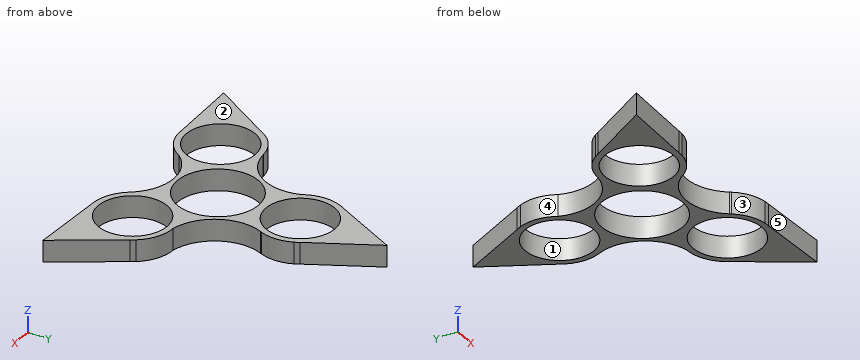
```python
from build123d import *

# Parameters (mm, degrees)
F0_R     = 11.2
F0_R_2   = 13.2
F1_DEPTH = 7


with BuildPart() as f1:
    # F0 (on Top) → F1 (new body)
    with BuildSketch(Plane.XY):
        with BuildLine():
            ThreePointArc((12.100793, 21.66292), (11.990187, 21.427431), (11.883555, 21.190116))
            ThreePointArc((11.883555, 21.190116), (11.994504, 21.425448), (12.100793, 21.66292))
        make_face()
        with BuildLine():
            ThreePointArc((23.327707, -0.268258), (12.397461, 7.683314), (11.883555, 21.190116))
            ThreePointArc((11.883555, 21.190116), (11.990187, 21.427431), (12.100793, 21.66292))
            ThreePointArc((12.100793, 21.66292), (13.199904, 26.986831), (12.060238, 32.302209))
            Line((12.060238, 32.302209), (11.254453, 33.834145))
            ThreePointArc((11.254453, 33.834145), (0, 40.136516), (-11.254453, 33.834145))
            Line((-11.254453, 33.834145), (-12.060238, 32.302209))
            ThreePointArc((-12.060238, 32.302209), (-13.181817, 26.243916), (-11.431535, 20.336516))
            ThreePointArc((-11.431535, 20.336516), (-12.852676, 6.894859), (-24.292957, -0.303597))
            ThreePointArc((-24.292957, -0.303597), (-24.551793, -0.329909), (-24.811035, -0.351866))
            ThreePointArc((-24.811035, -0.351866), (-29.971233, -2.061963), (-34.004652, -5.706632))
            Line((-34.004652, -5.706632), (-34.928456, -7.17043))
            ThreePointArc((-34.928456, -7.17043), (-34.759243, -20.068258), (-23.674002, -26.663715))
            Line((-23.674002, -26.663715), (-21.944414, -26.595577))
            ThreePointArc((-21.944414, -26.595577), (-16.136989, -24.537746), (-11.896172, -20.068258))
            ThreePointArc((-11.896172, -20.068258), (0.455215, -14.578173), (12.409401, -20.886519))
            ThreePointArc((12.409401, -20.886519), (12.561606, -21.097522), (12.710243, -21.311054))
            ThreePointArc((12.710243, -21.311054), (16.771329, -24.924868), (21.944414, -26.595577))
            Line((21.944414, -26.595577), (23.674002, -26.663715))
            ThreePointArc((23.674002, -26.663715), (34.759243, -20.068258), (34.928456, -7.17043))
            Line((34.928456, -7.17043), (34.004652, -5.706632))
            ThreePointArc((34.004652, -5.706632), (29.318806, -1.706169), (23.327707, -0.268258))
        make_face()
        with Locations((-23.327707, -13.468258)):
            Circle(F0_R, mode=Mode.SUBTRACT)
        with Locations((23.327707, -13.468258)):
            Circle(F0_R, mode=Mode.SUBTRACT)
        Circle(F0_R_2, mode=Mode.SUBTRACT)
        with Locations((0, 26.936516)):
            Circle(F0_R, mode=Mode.SUBTRACT)
        with BuildLine():
            Line((11.254453, 33.834145), (12.060238, 32.302209))
            ThreePointArc((12.060238, 32.302209), (11.682483, 33.081399), (11.254453, 33.834145))
        make_face()
        with BuildLine():
            ThreePointArc((34.928456, -7.17043), (34.490574, -6.423372), (34.004652, -5.706632))
            Line((34.004652, -5.706632), (34.928456, -7.17043))
        make_face()
        with BuildLine():
            ThreePointArc((-11.254453, 33.834145), (0, 40.136516), (11.254453, 33.834145))
            Line((11.254453, 33.834145), (0, 55.230804))
            Line((0, 55.230804), (-11.254453, 33.834145))
        make_face()
        with BuildLine():
            Line((47.831279, -27.615402), (34.928456, -7.17043))
            ThreePointArc((34.928456, -7.17043), (34.759243, -20.068258), (23.674002, -26.663715))
            Line((23.674002, -26.663715), (47.831279, -27.615402))
        make_face()
        with BuildLine():
            Line((-12.060238, 32.302209), (-11.254453, 33.834145))
            ThreePointArc((-11.254453, 33.834145), (-11.682483, 33.081399), (-12.060238, 32.302209))
        make_face()
        with BuildLine():
            ThreePointArc((21.944414, -26.595577), (22.80809, -26.658027), (23.674002, -26.663715))
            Line((23.674002, -26.663715), (21.944414, -26.595577))
        make_face()
        with BuildLine():
            ThreePointArc((12.409401, -20.886519), (12.55773, -21.100269), (12.710243, -21.311054))
            ThreePointArc((12.710243, -21.311054), (12.561606, -21.097522), (12.409401, -20.886519))
        make_face()
        with BuildLine():
            ThreePointArc((-24.811035, -0.351866), (-24.551793, -0.329909), (-24.292957, -0.303597))
            ThreePointArc((-24.292957, -0.303597), (-24.552234, -0.325179), (-24.811035, -0.351866))
        make_face()
        with BuildLine():
            Line((-34.928456, -7.17043), (-34.004652, -5.706632))
            ThreePointArc((-34.004652, -5.706632), (-34.490574, -6.423372), (-34.928456, -7.17043))
        make_face()
        with BuildLine():
            ThreePointArc((-23.674002, -26.663715), (-22.80809, -26.658027), (-21.944414, -26.595577))
            Line((-21.944414, -26.595577), (-23.674002, -26.663715))
        make_face()
        with BuildLine():
            ThreePointArc((-23.674002, -26.663715), (-34.759243, -20.068258), (-34.928456, -7.17043))
            Line((-34.928456, -7.17043), (-47.831279, -27.615402))
            Line((-47.831279, -27.615402), (-23.674002, -26.663715))
        make_face()
    extrude(amount=F1_DEPTH)


solid = f1.part
```
Could you check a few things on this model? Use its own coordinates, in mm. Face numbers are marked on the shaded views. A direction names the side the tool comes from. Coordinates: 2 decimals unless noted, no trailing zeros. Write each loop counter-clockwise with the first axis right and the second up, starting at its lowest first coordinate (ties: lowest second). Pieces come first, ordered by that corner, then holes. Notation, with made-up numbers: (22.5, 49.25) -> (44.5, 49.25) arc R13 ccw to (44.5, 58.25) -> close; hole circle Ø1 at (7.25, 79). An arc over 180 degrees is marked (long way). Write item = value, one per line. Start each with the question number.
(1) I want a section at A-A (x = -16.5). Please give me the cut outline in (y, z).
(2) I want a section at C-C (z = 4). Please give me the cut outline in (x, y).
(3) I need wall thicknesses on line 1 (X direction, y = -23.5, z = 5.5); line 2 (X direction, y = 20, z = 6.75); line 3 (X direction, y = 33, z = 4). Which ranges of each line are inside material? Lowest first, please. Write a range as [from, to].
(4) I want a section at B-B (y = 9). Please give me the cut outline in (x, z), plus the area to 3 significant figures.
(5) Which directions (+Z, -Z, +X, -X, +Y, -Y) give clear straight access to the entire face, cutting with the end or side of a thin tool? Please do the marked faces 4 and 5.
(6) We'd pull the mould along Y, two halves only. Please class the marked faces 1, 2 and 3: released by +Y, released by -Y, zero draft, split by the parting line, or undercut.
(7) Will these pins go through, and if not, where does the flat tip stop? pin 1 (1.5 mm diameter, centred on x = 35, z = 3.5, fed in from -Y); pin 2 (3 mm diameter, centred on x = 23.5, z = 3, fed in from +Y); pin 3 (2 mm diameter, centred on y = -1, z = 3, fed in from -X); pin 4 (13.5 mm diameter, centred on x = -23.33, y = -13.47, fed in from +Z).
(8) I want a section at D-D (x = -1.5). Please give me the cut outline in (y, z).
Result set:
q1.outline = (-24.77, 0) -> (-22.35, 0) -> (-22.35, 7) -> (-24.77, 7) -> close; (-4.59, 0) -> (2.85, 0) -> (2.85, 7) -> (-4.59, 7) -> close
q2.outline = (-47.83, -27.62) -> (-23.67, -26.66) arc R13.2 ccw to (-21.94, -26.6) arc R13.2 ccw to (-11.9, -20.07) arc R15.48 cw to (12.41, -20.89) arc R13.2 ccw to (12.71, -21.31) arc R13.2 ccw to (21.94, -26.6) arc R13.2 ccw to (23.67, -26.66) -> (47.83, -27.62) -> (34.93, -7.17) arc R13.2 ccw to (34, -5.71) arc R13.2 ccw to (23.33, -0.27) arc R15.48 cw to (11.88, 21.19) arc R13.2 ccw to (12.1, 21.66) arc R13.2 ccw to (12.06, 32.3) arc R13.2 ccw to (11.25, 33.83) -> (0, 55.23) -> (-11.25, 33.83) arc R13.2 ccw to (-12.06, 32.3) arc R13.2 ccw to (-11.43, 20.34) arc R15.48 cw to (-24.29, -0.3) arc R13.2 ccw to (-24.81, -0.35) arc R13.2 ccw to (-34, -5.71) arc R13.2 ccw to (-34.93, -7.17) -> close; hole circle Ø22.4 at (-23.33, -13.47); hole circle Ø26.4 at (0, 0); hole circle Ø22.4 at (0, 26.94); hole circle Ø22.4 at (23.33, -13.47)
q3.line_1 = [-45.23, -28.31], [-18.35, -14.75], [14.75, 18.35], [28.31, 45.23]
q3.line_2 = [-11.31, -8.79], [8.79, 11.42]
q3.line_3 = [-11.72, -9.42], [9.42, 11.72]
q4.outline = (-11.76, 0) -> (-9.66, 0) -> (-9.66, 7) -> (-11.76, 7) -> close; (9.66, 0) -> (11.77, 0) -> (11.77, 7) -> (9.66, 7) -> close
q4.area = 29.5 mm2
q5.face_4 = +Z, -Z, -X
q5.face_5 = +Z, -Z, -Y
q6.face_1 = undercut
q6.face_2 = zero draft
q6.face_3 = released by -Y
q7.pin_1 = -27.14
q7.pin_2 = 0.03
q7.pin_3 = -29.86
q7.pin_4 = through
q8.outline = (-14.64, 0) -> (-13.11, 0) -> (-13.11, 7) -> (-14.64, 7) -> close; (13.11, 0) -> (15.84, 0) -> (15.84, 7) -> (13.11, 7) -> close; (38.04, 0) -> (52.38, 0) -> (52.38, 7) -> (38.04, 7) -> close
